Work out the finished part from the listing and answer in its coordinate system (mm). Face numbers are marked on the shaded views. A direction names the side the tool comes from. Give positions to 0.01 mm unless a question says otherwise; leave off trailing zeros. Write each loop counter-clockwise with the first axis right and the second up, starting at its lowest first coordinate (ties: lowest second). Pieces come first, ordered by that corner, then holes.
1) Find section D-D (z = 6.25). Determine the outline of the cut face in (x, y).
2) A tool of negligible diameter and unlimited length cuts with its end or side. For the marked faces 1 and 2, from which of +Z, -Z, +X, -X, +Y, -Y can it reach the whole face along a straight path? Write none if from no direction.
3) Find section A-A (x = 0). Determine the outline of the cut face in (y, z), plus the area to 3 significant figures.
4) Determine the mould class of the marked faces 3, 4 and 5 for opening direction X: pulls with the +X half, pulls with the -X half, needs draft (parallel to the pull), parting line crosses it, or undercut.
5) Straight lines are drawn through the part: probe 1 along Y at (x, z) = (0, 5.25); probe 2 along X at (y, z) = (-12.5, 0.5); probe 3 along Z at (x, y) = (12.5, 23.5). For each, find the intervals that lie inside material, in ascending order.
6) Find section C-C (y = -6). Determine the outline of the cut face in (x, z), plus the area to 3 significant figures.
7) Given pin 1 Ø1 at (y, z) = (12.5, 0.5) entering from -X; pin 2 Ø0.6 at (x, z) = (5.5, 1) entering from -Y; pin 3 Ø1 at (y, z) = (-6, 0.5) entering from +X, each flat-ended and moving along its own axis, determine where each tip first touches the part or whether it passes through.
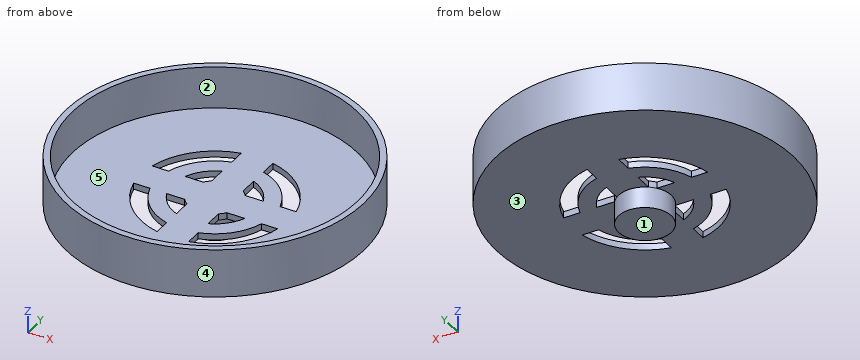
```python
from build123d import *

# Parameters (mm, degrees)
F0_R     = 28.2
F1_DEPTH = 9.2
F2_T     = -1.2
F4_DEPTH = 9.201
F5_R     = 5
F6_DEPTH = 4


# Not quite as in the source:
# - after a boolean that leaves OpenCascade's solid faulty, fix() repairs it


with BuildPart() as f1:
    # F0 (on Top) → F1 (new body)
    with BuildSketch(Plane.XY):
        Circle(F0_R)
    extrude(amount=F1_DEPTH)

    # F2
    f2_openings = [f1.faces().sort_by_distance(p)[0] for p in [
        (0, 0, 9.2),
    ]]
    offset(amount=F2_T, openings=f2_openings)

    # F3 (on face) → F4 (cut, through all)
    with BuildSketch(Plane(origin=(0, 0, 0), x_dir=(1, 0, 0), z_dir=(0, 0, -1))):
        with BuildLine():
            ThreePointArc((4, -3), (3.5355339059, -3.5355339059), (3, -4))
            Line((3, -4), (3, -7.4161984871))
            ThreePointArc((3, -7.4161984871), (5.6568542495, -5.6568542495), (7.4161984871, -3))
            Line((7.4161984871, -3), (4, -3))
        make_face()
        with BuildLine():
            ThreePointArc((10.5830052443, -3), (7.7781745931, -7.7781745931), (3, -10.5830052443))
            Line((3, -10.5830052443), (3, -13.6747943312))
            ThreePointArc((3, -13.6747943312), (9.8994949366, -9.8994949366), (13.6747943312, -3))
            Line((13.6747943312, -3), (10.5830052443, -3))
        make_face()
        with BuildLine():
            ThreePointArc((-13.6747943312, -3), (-9.8994949366, -9.8994949366), (-3, -13.6747943312))
            Line((-3, -13.6747943312), (-3, -10.5830052443))
            ThreePointArc((-3, -10.5830052443), (-7.7781745931, -7.7781745931), (-10.5830052443, -3))
            Line((-10.5830052443, -3), (-13.6747943312, -3))
        make_face()
        with BuildLine():
            ThreePointArc((-4, 3), (-3.5355339059, 3.5355339059), (-3, 4))
            Line((-3, 4), (-3, 7.4161984871))
            ThreePointArc((-3, 7.4161984871), (-5.6568542495, 5.6568542495), (-7.4161984871, 3))
            Line((-7.4161984871, 3), (-4, 3))
        make_face()
        with BuildLine():
            ThreePointArc((-10.5830052443, 3), (-7.7781745931, 7.7781745931), (-3, 10.5830052443))
            Line((-3, 10.5830052443), (-3, 13.6747943312))
            ThreePointArc((-3, 13.6747943312), (-9.8994949366, 9.8994949366), (-13.6747943312, 3))
            Line((-13.6747943312, 3), (-10.5830052443, 3))
        make_face()
        with BuildLine():
            Line((10.5830052443, 3), (13.6747943312, 3))
            ThreePointArc((13.6747943312, 3), (9.8994949366, 9.8994949366), (3, 13.6747943312))
            Line((3, 13.6747943312), (3, 10.5830052443))
            ThreePointArc((3, 10.5830052443), (7.7781745931, 7.7781745931), (10.5830052443, 3))
        make_face()
        with BuildLine():
            Line((4, 3), (7.4161984871, 3))
            ThreePointArc((7.4161984871, 3), (5.6568542495, 5.6568542495), (3, 7.4161984871))
            Line((3, 7.4161984871), (3, 4))
            ThreePointArc((3, 4), (3.5355339059, 3.5355339059), (4, 3))
        make_face()
        with BuildLine():
            Line((-4, -3), (-7.4161984871, -3))
            ThreePointArc((-7.4161984871, -3), (-5.6568542495, -5.6568542495), (-3, -7.4161984871))
            Line((-3, -7.4161984871), (-3, -4))
            ThreePointArc((-3, -4), (-3.5355339059, -3.5355339059), (-4, -3))
        make_face()
    extrude(amount=-F4_DEPTH, mode=Mode.SUBTRACT)

    # F5 (on face) → F6 (join)
    with BuildSketch(Plane(origin=(0, 0, 0), x_dir=(1, 0, 0), z_dir=(0, 0, -1))):
        Circle(F5_R)
    extrude(amount=F6_DEPTH)

    add(f1.part.fix(), mode=Mode.REPLACE)


solid = f1.part
```
Results:
1. outline: circle Ø56.4 at (0, 0); hole circle Ø54 at (0, 0)
2. face 1: -Z, +X, -X, +Y, -Y
2. face 2: +Z
3. outline: (-28.2, 0) - (-5, 0) - (-5, -4) - (5, -4) - (5, 0) - (28.2, 0) - (28.2, 9.2) - (27, 9.2) - (27, 1.2) - (-27, 1.2) - (-27, 9.2) - (-28.2, 9.2) - close
3. area: 127 mm2
4. face 3: needs draft
4. face 4: parting line crosses it
4. face 5: undercut
5. probe 1: y = -28.2 to -27, 27 to 28.2
5. probe 2: x = -25.28 to -6.3, -3 to 3, 6.3 to 25.28
5. probe 3: z = 0 to 1.2
6. outline: (-27.55, 0) - (-12.65, 0) - (-12.65, 1.2) - (-26.32, 1.2) - (-26.32, 9.2) - (-27.55, 9.2) - close; (-9.22, 0) - (-5.29, 0) - (-5.29, 1.2) - (-9.22, 1.2) - close; (-3, 0) - (3, 0) - (3, 1.2) - (-3, 1.2) - close; (5.29, 0) - (9.22, 0) - (9.22, 1.2) - (5.29, 1.2) - close; (12.65, 0) - (27.55, 0) - (27.55, 9.2) - (26.32, 9.2) - (26.32, 1.2) - (12.65, 1.2) - close
6. area: 72.1 mm2
7. pin 1: stops at x = -25.52
7. pin 2: stops at y = -27.72
7. pin 3: stops at x = 27.66
